from build123d import *

# Parameters (mm, degrees)
BOSS_EXTRUDE1_DEPTH = 0.5


with BuildPart() as part:
    # Model → Boss-Extrude1 (new body)
    with BuildSketch(Plane.XY):
        with BuildLine():
            Line((1535.049130397, 341.272822748), (1533.294327078, 341.272822748))
            ThreePointArc((1533.294327078, 341.272822748), (1533.044327078, 341.339810046), (1532.861314376, 341.522822748))
            Line((1532.861314376, 341.522822748), (1530.185887896, 346.156797344))
            ThreePointArc((1530.185887896, 346.156797344), (1530.135937685, 346.277387821), (1530.118900598, 346.406797344))
            Line((1530.118900598, 346.406797344), (1530.118900598, 351.772822748))
            ThreePointArc((1530.118900598, 351.772822748), (1529.53311416, 353.18703631), (1528.118900598, 353.772822748))
            Line((1528.118900598, 353.772822748), (1513.118900598, 353.772822748))
            ThreePointArc((1513.118900598, 353.772822748), (1511.704687035, 353.18703631), (1511.118900598, 351.772822748))
            Line((1511.118900598, 351.772822748), (1511.118900598, 346.406797344))
            ThreePointArc((1511.118900598, 346.406797344), (1511.101863511, 346.277387821), (1511.0519133, 346.156797344))
            Line((1511.0519133, 346.156797344), (1508.376486819, 341.522822748))
            ThreePointArc((1508.376486819, 341.522822748), (1508.193474117, 341.339810046), (1507.943474117, 341.272822748))
            Line((1507.943474117, 341.272822748), (1506.188670798, 341.272822748))
            ThreePointArc((1506.188670798, 341.272822748), (1505.90188258, 341.363246725), (1505.718824488, 341.601812676))
            Line((1505.718824488, 341.601812676), (1502.828165556, 349.543832819))
            ThreePointArc((1502.828165556, 349.543832819), (1502.645107463, 349.78239877), (1502.358319245, 349.872822748))
            Line((1502.358319245, 349.872822748), (1500.984812422, 349.872822748))
            ThreePointArc((1500.984812422, 349.872822748), (1500.734812422, 349.805835449), (1500.55179972, 349.622822748))
            Line((1500.55179972, 349.622822748), (1497.318638213, 344.022822748))
            ThreePointArc((1497.318638213, 344.022822748), (1497.135625511, 343.839810046), (1496.885625511, 343.772822748))
            Line((1496.885625511, 343.772822748), (1495.130822192, 343.772822748))
            ThreePointArc((1495.130822192, 343.772822748), (1494.844033974, 343.863246725), (1494.660975881, 344.101812676))
            Line((1494.660975881, 344.101812676), (1491.406346715, 353.043832819))
            ThreePointArc((1491.406346715, 353.043832819), (1491.223288623, 353.28239877), (1490.936500405, 353.372822748))
            Line((1490.936500405, 353.372822748), (1489.562993581, 353.372822748))
            ThreePointArc((1489.562993581, 353.372822748), (1489.312993581, 353.305835449), (1489.129980879, 353.122822748))
            Line((1489.129980879, 353.122822748), (1485.319469103, 346.522822748))
            ThreePointArc((1485.319469103, 346.522822748), (1485.136456401, 346.339810046), (1484.886456401, 346.272822748))
            Line((1484.886456401, 346.272822748), (1482.275131536, 346.272822748))
            ThreePointArc((1482.275131536, 346.272822748), (1481.921578145, 346.419269357), (1481.775131536, 346.772822748))
            Line((1481.775131536, 346.772822748), (1481.775131536, 365.772822748))
            ThreePointArc((1481.775131536, 365.772822748), (1481.921578145, 366.126376138), (1482.275131536, 366.272822748))
            Line((1482.275131536, 366.272822748), (1484.886456401, 366.272822748))
            ThreePointArc((1484.886456401, 366.272822748), (1485.136456401, 366.205835449), (1485.319469103, 366.022822748))
            Line((1485.319469103, 366.022822748), (1489.129980879, 359.422822748))
            ThreePointArc((1489.129980879, 359.422822748), (1489.312993581, 359.239810046), (1489.562993581, 359.172822748))
            Line((1489.562993581, 359.172822748), (1490.936500405, 359.172822748))
            ThreePointArc((1490.936500405, 359.172822748), (1491.223288623, 359.263246725), (1491.406346715, 359.501812676))
            Line((1491.406346715, 359.501812676), (1494.660975881, 368.443832819))
            ThreePointArc((1494.660975881, 368.443832819), (1494.844033974, 368.68239877), (1495.130822192, 368.772822748))
            Line((1495.130822192, 368.772822748), (1496.885625511, 368.772822748))
            ThreePointArc((1496.885625511, 368.772822748), (1497.135625511, 368.705835449), (1497.318638213, 368.522822748))
            Line((1497.318638213, 368.522822748), (1500.55179972, 362.922822748))
            ThreePointArc((1500.55179972, 362.922822748), (1500.734812422, 362.739810046), (1500.984812422, 362.672822748))
            Line((1500.984812422, 362.672822748), (1502.358319245, 362.672822748))
            ThreePointArc((1502.358319245, 362.672822748), (1502.645107463, 362.763246725), (1502.828165556, 363.001812676))
            Line((1502.828165556, 363.001812676), (1505.718824488, 370.943832819))
            ThreePointArc((1505.718824488, 370.943832819), (1505.90188258, 371.18239877), (1506.188670798, 371.272822748))
            Line((1506.188670798, 371.272822748), (1507.943474117, 371.272822748))
            ThreePointArc((1507.943474117, 371.272822748), (1508.193474117, 371.205835449), (1508.376486819, 371.022822748))
            Line((1508.376486819, 371.022822748), (1511.0519133, 366.388848151))
            ThreePointArc((1511.0519133, 366.388848151), (1511.101863511, 366.268257674), (1511.118900598, 366.138848151))
            Line((1511.118900598, 366.138848151), (1511.118900598, 360.772822748))
            ThreePointArc((1511.118900598, 360.772822748), (1511.704687035, 359.358609185), (1513.118900598, 358.772822748))
            Line((1513.118900598, 358.772822748), (1528.118900598, 358.772822748))
            ThreePointArc((1528.118900598, 358.772822748), (1529.53311416, 359.358609185), (1530.118900598, 360.772822748))
            Line((1530.118900598, 360.772822748), (1530.118900598, 366.138848151))
            ThreePointArc((1530.118900598, 366.138848151), (1530.135937685, 366.268257674), (1530.185887896, 366.388848151))
            Line((1530.185887896, 366.388848151), (1532.861314376, 371.022822748))
            ThreePointArc((1532.861314376, 371.022822748), (1533.044327078, 371.205835449), (1533.294327078, 371.272822748))
            Line((1533.294327078, 371.272822748), (1535.049130397, 371.272822748))
            ThreePointArc((1535.049130397, 371.272822748), (1535.335918615, 371.18239877), (1535.518976708, 370.943832819))
            Line((1535.518976708, 370.943832819), (1538.40963564, 363.001812676))
            ThreePointArc((1538.40963564, 363.001812676), (1538.592693732, 362.763246725), (1538.87948195, 362.672822748))
            Line((1538.87948195, 362.672822748), (1540.252988773, 362.672822748))
            ThreePointArc((1540.252988773, 362.672822748), (1540.502988773, 362.739810046), (1540.686001475, 362.922822748))
            Line((1540.686001475, 362.922822748), (1543.919162983, 368.522822748))
            ThreePointArc((1543.919162983, 368.522822748), (1544.102175685, 368.705835449), (1544.352175685, 368.772822748))
            Line((1544.352175685, 368.772822748), (1546.106979004, 368.772822748))
            ThreePointArc((1546.106979004, 368.772822748), (1546.393767222, 368.68239877), (1546.576825314, 368.443832819))
            Line((1546.576825314, 368.443832819), (1549.831454481, 359.501812676))
            ThreePointArc((1549.831454481, 359.501812676), (1550.014512573, 359.263246725), (1550.301300791, 359.172822748))
            Line((1550.301300791, 359.172822748), (1551.674807614, 359.172822748))
            ThreePointArc((1551.674807614, 359.172822748), (1551.924807614, 359.239810046), (1552.107820316, 359.422822748))
            Line((1552.107820316, 359.422822748), (1555.918332093, 366.022822748))
            ThreePointArc((1555.918332093, 366.022822748), (1556.101344795, 366.205835449), (1556.351344795, 366.272822748))
            Line((1556.351344795, 366.272822748), (1558.96266966, 366.272822748))
            ThreePointArc((1558.96266966, 366.272822748), (1559.316223051, 366.126376138), (1559.46266966, 365.772822748))
            Line((1559.46266966, 365.772822748), (1559.46266966, 346.772822748))
            ThreePointArc((1559.46266966, 346.772822748), (1559.316223051, 346.419269357), (1558.96266966, 346.272822748))
            Line((1558.96266966, 346.272822748), (1556.351344795, 346.272822748))
            ThreePointArc((1556.351344795, 346.272822748), (1556.101344795, 346.339810046), (1555.918332093, 346.522822748))
            Line((1555.918332093, 346.522822748), (1552.107820316, 353.122822748))
            ThreePointArc((1552.107820316, 353.122822748), (1551.924807614, 353.305835449), (1551.674807614, 353.372822748))
            Line((1551.674807614, 353.372822748), (1550.301300791, 353.372822748))
            ThreePointArc((1550.301300791, 353.372822748), (1550.014512573, 353.28239877), (1549.831454481, 353.043832819))
            Line((1549.831454481, 353.043832819), (1546.576825314, 344.101812676))
            ThreePointArc((1546.576825314, 344.101812676), (1546.393767222, 343.863246725), (1546.106979004, 343.772822748))
            Line((1546.106979004, 343.772822748), (1544.352175685, 343.772822748))
            ThreePointArc((1544.352175685, 343.772822748), (1544.102175685, 343.839810046), (1543.919162983, 344.022822748))
            Line((1543.919162983, 344.022822748), (1540.686001475, 349.622822748))
            ThreePointArc((1540.686001475, 349.622822748), (1540.502988773, 349.805835449), (1540.252988773, 349.872822748))
            Line((1540.252988773, 349.872822748), (1538.87948195, 349.872822748))
            ThreePointArc((1538.87948195, 349.872822748), (1538.592693732, 349.78239877), (1538.40963564, 349.543832819))
            Line((1538.40963564, 349.543832819), (1535.518976708, 341.601812676))
            ThreePointArc((1535.518976708, 341.601812676), (1535.335918616, 341.363246725), (1535.049130397, 341.272822748))
        make_face()
    extrude(amount=BOSS_EXTRUDE1_DEPTH)


solid = part.part
For this review, take the finished solid that the model builds, in its own axes (mm). A direction names the side the tool comes from. Coordinates: 2 decimals unless noted, no trailing zeros. Order: outer loops, then holes, each group sorted by start corner. A loop starts at its lowest first (then second) coordinate and runs counter-clockwise, first axis right, second up. Notation, with made-up numbers: (84.5, 53.25) - (103.5, 53.25) arc R24 cw to (103.5, 80.25) - close; hole circle Ø6 at (45, 46.5). An arc over 180 degrees is marked (long way). Use one line per item in the form item = value.
Q1. For faces 1 (the flat face through (1521, 356, 0.5)), 2 (the flat face through (1531.505, 368.673, 0.246)), 3 (the flat face through (1542.325, 346.784, 0.246)), list the 3-axis set-ups (+Z, -Z, +X, -X, +Y, -Y) from which the entire face can be reached by the end or side of a thin tool; tool diameter is ignored.
Checked values:
face_1 = +Z, +X, -X, +Y, -Y
face_2 = +Z, -Z, +Y
face_3 = +Z, -Z, -Y
Q2. Consider section B-B (x = 1514). Give the boundary of the cut face in (y, z).
Checked values:
outline = (353.77, 0) - (358.77, 0) - (358.77, 0.5) - (353.77, 0.5) - close
Q3. For P1, Ø1, axis at x = 1515, y = 355.5, coming from the -Z side, flat-tipped, find the tip position at first contact; note if it passes through.
Checked values:
P1 = 0
Q4. Consider section A-A (y = 367.5). Give the boundary of the cut face in (x, z), then the cut area to 3 significant figures.
Checked values:
outline = (1494.32, 0) - (1497.91, 0) - (1497.91, 0.5) - (1494.32, 0.5) - close; (1504.47, 0) - (1510.41, 0) - (1510.41, 0.5) - (1504.47, 0.5) - close; (1530.83, 0) - (1536.77, 0) - (1536.77, 0.5) - (1530.83, 0.5) - close; (1543.33, 0) - (1546.92, 0) - (1546.92, 0.5) - (1543.33, 0.5) - close
area = 9.54 mm2
Q5. Draft analysis for pull direction X (two halves, no side actions). For faces 4 (the flat face through (1521, 356, 0)), 5 (the flat face through (1493.056, 348.51, 0.246)), state which applies: +X half, -X half, draft (parallel to the pull), parting line (faces both ways), or undercut.
Checked values:
face_4 = draft
face_5 = undercut
Q6. Consider section C-C (x = 1536.5). Give the boundary of the cut face in (y, z).
Checked values:
outline = (344.3, 0) - (368.25, 0) - (368.25, 0.5) - (344.3, 0.5) - close
Q7. For probe 1 along X at (y, z) = (362, 0.3); probe 2 along X at (y, z) = (346, 0.35); probe 3 along X at (y, z) = (364, 0.4), list the stretches that pass through material, from the lowest coordinate up. Write a range as from..to.
Checked values:
probe_1 = 1481.78..1487.64, 1492.32..1511.12, 1530.12..1548.92, 1553.6..1559.46
probe_2 = 1493.97..1498.46, 1504.12..1510.96, 1530.28..1537.12, 1542.78..1547.27
probe_3 = 1481.78..1486.49, 1493.04..1499.93, 1503.19..1511.12, 1530.12..1538.05, 1541.31..1548.19, 1554.75..1559.46
